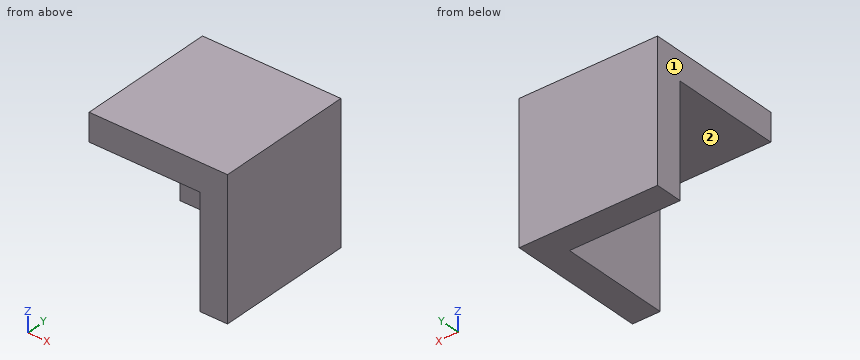
```python
from build123d import *

# Parameters (mm, degrees)
BOX_W        = 10
BOX_H        = 10
BOX_DEPTH    = 10
BOX001_W     = 10
BOX001_H     = 10
BOX001_DEPTH = 10


with BuildPart() as cub_base:
    # Box → Box (new body)
    with BuildSketch(Plane.XY):
        with Locations((5, 5)):
            Rectangle(BOX_W, BOX_H)
    extrude(amount=BOX_DEPTH)


with BuildPart() as cut:
    # Box001 → Box001 (new body)
    with BuildSketch(Plane(origin=(2, 2, 2), x_dir=(1, 0, 0), z_dir=(0, 0, 1))):
        with Locations((5, 5)):
            Rectangle(BOX001_W, BOX001_H)
    extrude(amount=BOX001_DEPTH)

    # Cut: cut Cub-Base
    add(cub_base.part, mode=Mode.SUBTRACT)


solid = cut.part
```
Here's how the part is built. I have some questions about the finished solid (model axes, mm). Face numbers are marked on the shaded views. A direction names the side the tool comes from. Round coordinates to 2 decimals unless told otherwise and drop trailing zeros. Order: outer loops, then holes, each group sorted by start corner. A loop starts at its lowest first (then second) coordinate and runs counter-clockwise, first axis right, second up. Notation, with made-up numbers: M 69.5,23.5 L 82.5,23.5 A35 ccw 82.5,58.5 Z; hole C 36.25,76 d5. An arc over 180 degrees is marked long. Use CSV: the item, a comma, the result in double quotes.
1) I'm going to push flat-ended pins straight in: P1, Ø3, axis at x = 7, y = 7, coming from the -Z side; P2, Ø2, axis at x = 5.5, z = 5.5, coming from the -Y side; P3, Ø2.5, axis at y = 8, z = 8, coming from the -X side. Where does each tip first touch, or does it pass through?
Taken from the geometry:
P1,"z = 10"
P2,"y = 10"
P3,"x = 10"
2) I need wall thicknesses on line 1 along Z through (x, y) = (7, 5.25). Which ranges of the line are inside material? Lowest first, please. Write a range as [from, to].
Taken from the geometry:
line 1,"[10, 12]"
3) On a 3-axis mill with a long thin cutter (end or side, diameter ignored), from which of +Z, -Z, +X, -X, +Y, -Y can I reach the whole of each face in a straight line? I mean the marked faces 1 and 2. Say none if no direction works.
Taken from the geometry:
face 1,"+Z, -Z, -X, +Y, -Y"
face 2,"-Z, -X, -Y"
4) I want a section at A-A (z = 9.75). List the corners of the cut face in (x, y) for me.
Taken from the geometry:
outline,"M 2,10 L 10,10 L 10,2 L 12,2 L 12,12 L 2,12 Z"
